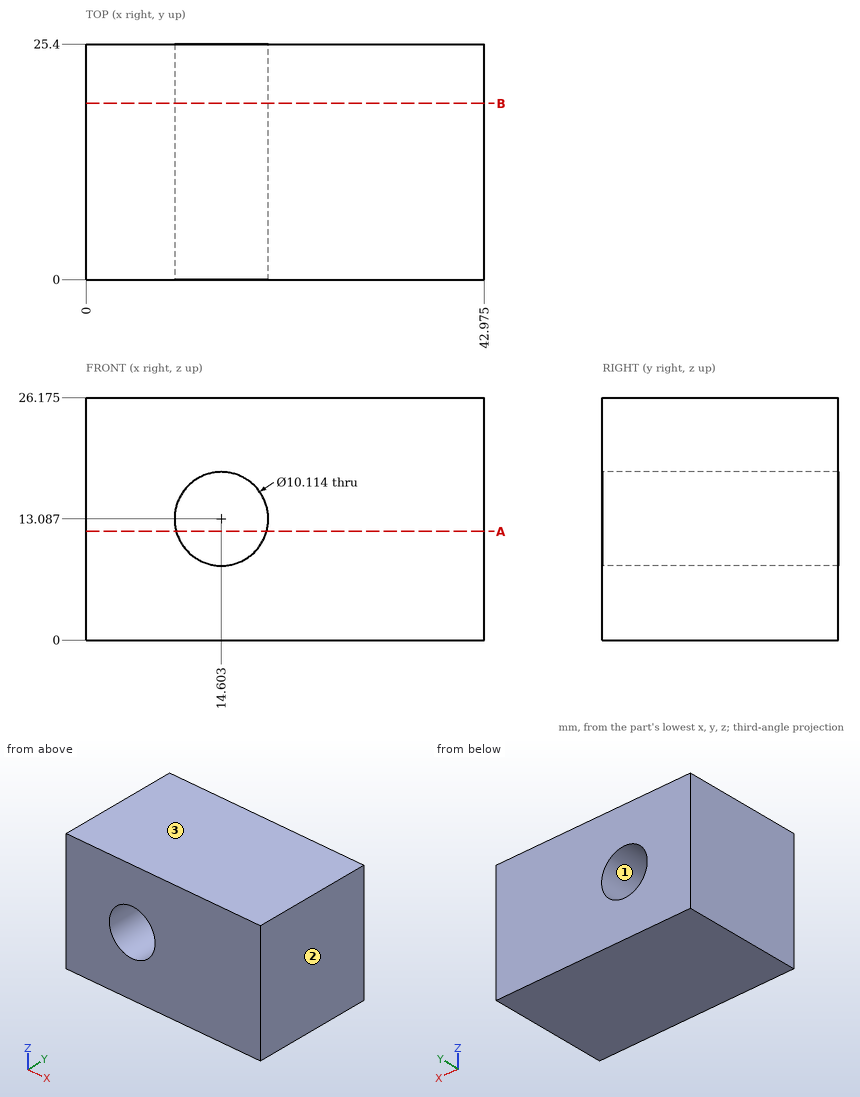
The drawing under review shows one solid part. Ordinate dimensions are in mm from its lowest x, y, z. Round coordinates to 2 decimals unless told otherwise and drop trailing zeros. Write each loop counter-clockwise with the first axis right and the second up, starting at its lowest first coordinate (ties: lowest second). Pieces come first, ordered by that corner, then holes. Notation, with made-up numbers: (25.5, 52.5) -> (35.5, 52.5) arc R29 ccw to (35.5, 91.5) -> close; hole circle Ø11 at (13, 60.25). An arc over 180 degrees is marked (long way). Put each result on its own line as item: value.
Q1. To check wall thickness, follow L1, parallel to X at y = 5.5, z = 13 (1 decimal); L2, parallel to Z at x = 16.5, y = 3 (1 decimal); L3, parallel to X at y = 5, z = 10.75 (1 decimal). State the ranges of each line that lie inside material, in increasing order. Write a range as [from, to].
Determined:
L1: x = [0, 9.5], [19.7, 43]
L2: z = [0, 8.4], [17.8, 26.2]
L3: x = [0, 10.1], [19.1, 43]
Q2. Consider section B-B on y = 19. State the section outline as (x, z) points (1 decimal).
Determined:
outline: (0, 0) -> (43, 0) -> (43, 26.2) -> (0, 26.2) -> close; hole circle Ø10.1 at (14.6, 13.1)
Q3. The part is to be moulded in two halves that separate along Z. For the marked faces 1, 2 and 3, say which applies: released by +Z, released by -Z, zero draft, split by the parting line, or undercut.
Determined:
face 1: undercut
face 2: zero draft
face 3: released by +Z
Q4. Consider section A-A on z = 11.75. State the section outline as (x, y) points (1 decimal).
Determined:
outline: (0, 0) -> (9.7, 0) -> (9.7, 25.4) -> (0, 25.4) -> close; (19.5, 0) -> (43, 0) -> (43, 25.4) -> (19.5, 25.4) -> close
